Autodesk Inventor part; units mm, degrees
ref_plane "РабПлоскость1" through (0, 0, 40) normal (0, 0, 1) x (1, 0, 0)
ref_plane "РабПлоскость2" through (0, 0, 50) normal (0, 0, 1) x (1, 0, 0)
ref_plane "РабПлоскость3" through (-5, 0, 40) normal (1, 0, 0) x (0, 1, 0)
sketch "Эскиз1" plane through (0, 0, 0) normal (0, 0, 1) x (1, 0, 0)
  circle A0 centre (0, 0) radius 3
  dimension "d0" = 6
extrude "Выдавливание1" add sketch "Эскиз1" along normal blind 40
ref_plane "РабПлоскость1" through (0, 0, 40) normal (0, 0, 1) x (1, 0, 0)
sketch "Эскиз2" plane through (0, 0, 40) normal (0, 0, 1) x (1, 0, 0)
  circle A0 centre (0, 0) radius 5
  dimension "d4" = 10
extrude "Выдавливание2" add sketch "Эскиз2" along normal blind 10
ref_plane "РабПлоскость2" through (0, 0, 50) normal (0, 0, 1) x (1, 0, 0)
sketch "Эскиз3" plane through (0, 0, 50) normal (0, 0, 1) x (1, 0, 0)
  line L0 (-2, 8) -> (2, 8)
  line L1 (2, 8) -> (2, -7)
  line L2 (2, -7) -> (-2, -7)
  line L3 (-2, -7) -> (-2, 8)
  point P0 (0, 0)
  dimension "d8" = 4
  dimension "d9" = 15
extrude "Выдавливание3" cut sketch "Эскиз3" against normal blind 8
ref_plane "РабПлоскость3" through (-5, 0, 40) normal (1, 0, 0) x (0, 1, 0)
sketch "Эскиз4" plane through (-5, 0, 40) normal (1, 0, 0) x (0, 1, 0)
  circle A0 centre (0, 6) radius 1.5
  line L0 (4.5826, 10) -> (-4.5826, 10)
  point P0 (0, -40)
  dimension "d12" = 3
  dimension "d13" = 4
extrude "Выдавливание4" cut sketch "Эскиз4" along normal blind 10
ref_plane "РабПлоскость4" through (0, 0, 0) normal (0, 0, -1) x (-1, 0, 0)
sketch "Эскиз5" plane through (0, 0, 0) normal (0, 0, -1) x (-1, 0, 0)
  circle A0 centre (0, 0) radius 2
  dimension "d17" = 4
extrude "Выдавливание5" add sketch "Эскиз5" along normal blind 1.5
ref_plane "РабПлоскость5" through (0, 0, -1.5) normal (0, 0, -1) x (-1, 0, 0)
sketch "Эскиз6" plane through (0, 0, -1.5) normal (0, 0, -1) x (-1, 0, 0)
  circle A0 centre (0, 0) radius 2.5
  dimension "d21" = 5
extrude "Выдавливание6" add sketch "Эскиз6" along normal blind 1
chamfer "Фаска1" distance 1 angle 45 1 edges at (-5, 0, 40)
thread "Резьба1"
properties part number "крепёж"
The model under review builds one solid part; all positions refer to its coordinate system, in mm. A direction names the side the tool comes from. Coordinates: 2 decimals unless noted, no trailing zeros. Write each loop counter-clockwise with the first axis right and the second up, starting at its lowest first coordinate (ties: lowest second). Pieces come first, ordered by that corner, then holes. Notation, with made-up numbers: M 83,-26.75 L 118,-26.75 A28 ccw 118,-1.75 Z; hole C 53,59.5 d2. An arc over 180 degrees is marked long. Put each result on its own line as item: value.
1) Add section C-C on z = 46. Give the boundary of the cut face in (x, y), then the cut area to 3 significant figures.
Computed:
outline: M -4.77,-1.5 A5 ccw -2,-4.58 L -2,-1.5 Z; M -4.77,1.5 L -2,1.5 L -2,4.58 A5 ccw Z; M 2,-4.58 A5 ccw 4.77,-1.5 L 2,-1.5 Z; M 2,1.5 L 4.77,1.5 A5 ccw 2,4.58 Z
area: 22.1 mm2
2) For faces 1 (the flat face through (0, 0, 42)), 2 (the cylindrical face through (3.48, -1.5, 45.93)), 3 (the cylindrical face through (0, 2, -1)), 4 (the cylindrical face through (0.54, 2.44, -1.99)), list the 3-axis set-ups (+Z, -Z, +X, -X, +Y, -Y) from which the entire face can be reached by the end or side of a thin tool; tool diameter is ignored.
Computed:
face 1: +Z, +Y, -Y
face 2: +X, -X
face 3: none
face 4: -Z
3) Add section A-A on y = 0. State how many separate pieces and enclosed holes the cut face has, then the cut area to 3 significant figures.
Computed:
separate pieces: 3
enclosed holes: 0
area: 300 mm2
4) Wall thickness on probe 1 along Z at (x, y) = (2.95, 0); probe 2 along Z at (x, y) = (1, 3.75); probe 3 along Y at (x, z) = (-3, 44): over which ranges is each line inside the solid? List them lowest first. Write a range as [from, to].
Computed:
probe 1: z = [0, 44.5], [47.5, 50]
probe 2: z = [40, 42]
probe 3: y = [-4, 4]
5) Draft analysis for pull direction Z (two halves, no side actions). For faces 5 (the flat face through (-2, 0, 44)), 6 (the flat face through (3, 0, 50)), 7 (the flat face through (1, -2, 0)), state which applies: released by +Z, released by -Z, zero draft, split by the parting line, or undercut.
Computed:
face 5: zero draft
face 6: released by +Z
face 7: undercut
6) Add section B-B on x = 0. Give the boundary of the cut face in (y, z), then the cut area to 3 significant figures.
Computed:
outline: M -5,41 L -4,40 L -3,40 L -3,0 L -2,0 L -2,-1.5 L -2.5,-1.5 L -2.5,-2.5 L 2.5,-2.5 L 2.5,-1.5 L 2,-1.5 L 2,0 L 3,0 L 3,40 L 4,40 L 5,41 L 5,42 L -5,42 Z
area: 270 mm2
7) Clearance check with flat-ended pins moving along their axes: pin 1 Ø1.5 at (x, z) = (-0.5, 8) entering from -Y; pin 2 Ø1 at (y, z) = (1, 32) entering from +X; pin 3 Ø1 at (y, z) = (2.5, 3) entering from -X. State where each tip first meets the part, or that it passes through.
Computed:
pin 1: stops at y = -3
pin 2: stops at x = 2.96
pin 3: stops at x = -2.24
8) Add section D-D on z = 39. Give the boundary of the cut face in (x, y).
Computed:
outline: C 0,0 d6
